Geometry: final body of the model. Coordinates: model frame, mm. Round coordinates to 2 decimals unless told otherwise and drop trailing zeros. Loops run counter-clockwise (first coordinate to the right, second up) from the corner with the lowest first, then second, coordinate; pieces in that order, holes last. Notation, with made-up numbers: M 63.25,65 L 110.25,65 A19 cw 110.25,97 Z; hole C -17,21 d3. An arc over 180 degrees is marked long. Answer as a JSON object with one key per item and string values.
```python
from build123d import *

# Parameters (mm, degrees)
SKETCH_1_R      = 1.45
EXTRUDE_1_DEPTH = 3
FILLET_1_R      = 5


with BuildPart() as part:
    # 草图1 → 凸台-拉伸1 (new body)
    with BuildSketch(Plane(origin=(0, 0, 0), x_dir=(1, 0, 0), z_dir=(0, 1, 0))):
        Polygon((0, 0), (0, -10), (-1.089249024, -24.960398944), (18.857949568, -26.412730977), (19.947198592, -11.452332033), (20.781029397, 0), (32, 0), (32, 15), (20.781029397, 15), (0, 15), align=None)
        with Locations(Location((5, 7.5, 0), (0, 0, 270))):
            Circle(SKETCH_1_R, mode=Mode.SUBTRACT)
        with Locations(Location((22, 7.5, 0), (0, 0, 270))):
            Circle(SKETCH_1_R, mode=Mode.SUBTRACT)
        with Locations(Location((4.442175136, -17.84328248, 0), (0, 0, 270))):
            Circle(SKETCH_1_R, mode=Mode.SUBTRACT)
        with Locations(Location((14.415774432, -18.569448496, 0), (0, 0, 270))):
            Circle(SKETCH_1_R, mode=Mode.SUBTRACT)
        with Locations(Location((5, -5, 0), (0, 0, 270))):
            Circle(SKETCH_1_R, mode=Mode.SUBTRACT)
        with Locations(Location((15, -5, 0), (0, 0, 270))):
            Circle(SKETCH_1_R, mode=Mode.SUBTRACT)
    extrude(amount=EXTRUDE_1_DEPTH)

    # 圆角1
    # the kernel refuses this fillet: 5 mm, written as the material it adds along each edge
    with BuildSketch(Plane(origin=(20.781029397, 0, 0), x_dir=(1, 0, 0), z_dir=(0, 1, 0))) as fillet_1_piece_1:
        with BuildLine():
            CenterArc((FILLET_1_R * 0.929838236779, -FILLET_1_R), FILLET_1_R, 90, 85.835709886)
            Line((-FILLET_1_R * 0.0675216928189, -FILLET_1_R * 0.927383398372), (0, 0))
            Line((0, 0), (FILLET_1_R * 0.929838236779, 0))
        make_face()
    extrude(amount=3)
    with BuildSketch(Plane(origin=(0, 0, 10), x_dir=(0, 0, -1), z_dir=(0, 1, 0))) as fillet_1_piece_2:
        with BuildLine():
            CenterArc((FILLET_1_R * 0.0363562923998, FILLET_1_R), FILLET_1_R, 265.835709886, 4.164290114)
            Line((-FILLET_1_R * 0.0362603092284, FILLET_1_R * 0.00264007040188), (0, 0))
            Line((0, 0), (FILLET_1_R * 0.0363562923998, 0))
        make_face()
    extrude(amount=3)
    # the kernel refuses this fillet: 5 mm, written as the material it takes off along each edge
    with BuildSketch(Plane(origin=(0, -12.5, -15), x_dir=(0, 0, 1), z_dir=(0, 1, 0)), Plane(origin=(32, -12.5, -15), x_dir=(-1, 0, 0), z_dir=(0, 1, 0))) as fillet_1_2_piece_1:
        with BuildLine():
            CenterArc((FILLET_1_R, FILLET_1_R), FILLET_1_R, 180, 90)
            Line((0, FILLET_1_R), (0, 0))
            Line((0, 0), (FILLET_1_R, 0))
        make_face()
    extrude(amount=28, mode=Mode.SUBTRACT)
    with BuildSketch(Plane(origin=(32, -12.5, 0), x_dir=(-1, 0, 0), z_dir=(0, 1, 0)), Plane(origin=(18.857949568, -12.5, 26.412730977), x_dir=(-0.9973599295981169, 0, -0.0726166016282719), z_dir=(0, 1, 0)), Plane(origin=(-1.089249024, -12.5, 24.960398944), x_dir=(0.07261660162819664, 0, -0.9973599295981225), z_dir=(0, 1, 0))) as fillet_1_2_piece_2:
        with BuildLine():
            CenterArc((FILLET_1_R, -FILLET_1_R), FILLET_1_R, 90, 90)
            Line((0, -FILLET_1_R), (0, 0))
            Line((0, 0), (FILLET_1_R, 0))
        make_face()
    extrude(amount=28, mode=Mode.SUBTRACT)


solid = part.part
```
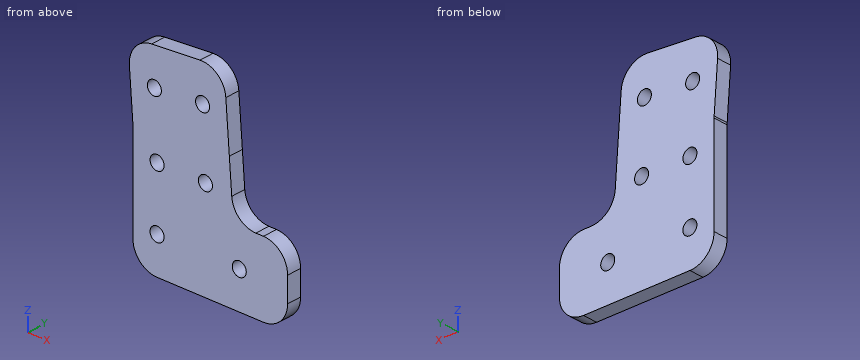
1) Cut plane A-A on z = -7.5. Return the cut outline in (x, y), and give its area (3 significant figures).
Geometry results:
{"outline": "M 0,0 L 3.55,0 L 3.55,3 L 0,3 Z; M 6.45,0 L 20.55,0 L 20.55,3 L 6.45,3 Z; M 23.45,0 L 32,0 L 32,3 L 23.45,3 Z", "area": "78.6 mm2"}
2) First-contact query: pin 1 (2.5 mm diameter, centred on x = 5, z = -7.5, fed in from -Y); pin 2 (4 mm diameter, centred on x = 15, z = 5, fed in from +Y); pin 3 (0.9 mm diameter, centred on y = 1, z = -1, fed in from -X); pin 4 (0.5 mm diameter, centred on x = 26.5, y = 2, fed in from +Z). Flat tips, straight axial feed; report the tip coordinate or a pass-through.
Geometry results:
{"pin 1": "through", "pin 2": "y = 3", "pin 3": "x = 0", "pin 4": "z = 0"}
3) Cut plane D-D on x = 22. Return the cut outline in (y, z), and give its area (3 significant figures).
Geometry results:
{"outline": "M 0,-15 L 3,-15 L 3,-8.95 L 0,-8.95 Z; M 0,-6.05 L 3,-6.05 L 3,1.36 L 0,1.36 Z", "area": "40.4 mm2"}
4) Line query: probe 1 along X at (y, z) = (1.35, -7.5); probe 2 along X at (y, z) = (0.95, 5); probe 3 along Z at (x, y) = (14.5, 1.2). Output: solid intervals per line, ascending.
Geometry results:
{"probe 1": "0 to 3.55, 6.45 to 20.55, 23.45 to 32", "probe 2": "0 to 3.55, 6.45 to 13.55, 16.45 to 20.42", "probe 3": "-15 to 3.64, 6.36 to 17.12, 20.02 to 26.06"}
5) Cut plane C-C on y = 2.5. Return the cut outline in (x, z), and give its area (3 significant figures).
Geometry results:
{"outline": "M -0.73,19.97 L -0.01,10.18 A5 cw 0,9.82 L 0,-10 A5 ccw 5,-15 L 27,-15 A5 ccw 32,-10 L 32,-5 A5 ccw 27,0 L 25.43,0 A5 cw 20.44,4.64 L 19.22,21.43 A5 ccw 13.87,26.05 L 3.9,25.32 A5 ccw Z; hole C 4.44,17.84 d2.9; hole C 5,-7.5 d2.9; hole C 5,5 d2.9; hole C 14.42,18.57 d2.9; hole C 15,5 d2.9; hole C 22,-7.5 d2.9", "area": "937 mm2"}
6) Cut plane B-B on x = 15. Return the cut outline in (y, z), and give its area (3 significant figures).
Geometry results:
{"outline": "M 0,-15 L 3,-15 L 3,3.55 L 0,3.55 Z; M 0,6.45 L 3,6.45 L 3,17.24 L 0,17.24 Z; M 0,19.9 L 3,19.9 L 3,26 L 0,26 Z", "area": "106 mm2"}
